```python
from build123d import *

# Parameters (mm, degrees)
BOSS_EXTRUDE1_DEPTH = 4.5
FILLET1_R           = 0.3
FILLET2_R           = 0.3
SHELL3_START        = 0.35
SHELL3_DEPTH        = 3.8
SKETCH3_W           = 12.9
SKETCH3_H           = 3.9
CUT_EXTRUDE1_DEPTH  = 21
CUT_EXTRUDE2_REACH  = 27.289
SKETCH4_W           = 3
SKETCH4_H           = 2.5


# Read off the part's stored shape, not the designer's step: Shell3
with BuildPart() as part:
    # Sketch1 → Boss-Extrude1 (new body)
    with BuildSketch(Plane(origin=(0, 0, 0), x_dir=(1, 0, 0), z_dir=(0, 1, 0))):
        Polygon((-6.75, -7.047619048), (6.75, -7.047619048), (6.75, 13.952380952), (6, 15.365710355), (6, 23.952380952), (-6, 23.952380952), (-6, 15.365710355), (-6.75, 13.952380952), align=None)
    extrude(amount=BOSS_EXTRUDE1_DEPTH)

    # Fillet1
    fillet1_edges = [part.edges().sort_by_distance(p)[0] for p in [
        (6, 4.5, -19.659045654),
        (6.375, 0, -14.659045654),
        (6.75, 0, -3.452380952),
        (0, 4.5, -23.952380952),
        (-6, 4.5, -19.659045654),
        (-6.375, 4.5, -14.659045654),
        (-6.75, 4.5, -3.452380952),
        (0, 4.5, 7.047619048),
        (6.75, 4.5, -3.452380952),
        (6.375, 4.5, -14.659045654),
        (0, 0, 7.047619048),
        (-6.75, 0, -3.452380952),
        (-6.375, 0, -14.659045654),
        (-6, 0, -19.659045654),
        (0, 0, -23.952380952),
        (6, 0, -19.659045654),
    ]]
    fillet(fillet1_edges, radius=FILLET1_R)

    # Fillet2
    # the kernel refuses this fillet: 0.3 mm, written as the material it takes off along each edge
    with BuildSketch(Plane(origin=(-6.45, 0.3, 6.747619048), x_dir=(-1, 0, 0), z_dir=(0, 0, 1))) as fillet2_piece_1_section:
        Polygon((0, 0), (FILLET2_R, 0), (FILLET2_R, FILLET2_R), (0, FILLET2_R), align=None)
    fillet2_piece_1 = extrude(amount=FILLET2_R, mode=Mode.PRIVATE)
    fillet2_piece_1 = fillet2_piece_1 - Plane(origin=(-6.45, 0.3, 6.747619048), x_dir=(0.7071067811865475, 0.7071067811865475, 0), z_dir=(0, 0, 1)) * Sphere(FILLET2_R, mode=Mode.PRIVATE)
    add(fillet2_piece_1, mode=Mode.SUBTRACT)
    with BuildSketch(Plane(origin=(-5.7, 0.3, -23.652380952), x_dir=(0, 0, -1), z_dir=(-1, 0, 0))) as fillet2_piece_2_section:
        Polygon((0, 0), (FILLET2_R, 0), (FILLET2_R, FILLET2_R), (0, FILLET2_R), align=None)
    fillet2_piece_2 = extrude(amount=FILLET2_R, mode=Mode.PRIVATE)
    fillet2_piece_2 = fillet2_piece_2 - Plane(origin=(-5.7, 0.3, -23.652380952), x_dir=(0, 0.7071067811865475, 0.7071067811865475), z_dir=(-1, 0, 0)) * Sphere(FILLET2_R, mode=Mode.PRIVATE)
    add(fillet2_piece_2, mode=Mode.SUBTRACT)
    with BuildSketch(Plane(origin=(6.45, 0.3, 6.747619048), x_dir=(1, 0, 0), z_dir=(0, 0, 1))) as fillet2_piece_3_section:
        Polygon((0, 0), (FILLET2_R, 0), (FILLET2_R, -FILLET2_R), (0, -FILLET2_R), align=None)
    fillet2_piece_3 = extrude(amount=FILLET2_R, mode=Mode.PRIVATE)
    fillet2_piece_3 = fillet2_piece_3 - Plane(origin=(6.45, 0.3, 6.747619048), x_dir=(-0.7071067811865475, 0.7071067811865475, 0), z_dir=(0, 0, 1)) * Sphere(FILLET2_R, mode=Mode.PRIVATE)
    add(fillet2_piece_3, mode=Mode.SUBTRACT)
    with BuildSketch(Plane(origin=(5.7, 0.3, -23.652380952), x_dir=(0, 0, -1), z_dir=(1, 0, 0))) as fillet2_piece_4_section:
        Polygon((0, 0), (FILLET2_R, 0), (FILLET2_R, -FILLET2_R), (0, -FILLET2_R), align=None)
    fillet2_piece_4 = extrude(amount=FILLET2_R, mode=Mode.PRIVATE)
    fillet2_piece_4 = fillet2_piece_4 - Plane(origin=(5.7, 0.3, -23.652380952), x_dir=(0, 0.7071067811865475, 0.7071067811865475), z_dir=(1, 0, 0)) * Sphere(FILLET2_R, mode=Mode.PRIVATE)
    add(fillet2_piece_4, mode=Mode.SUBTRACT)
    with BuildSketch(Plane(origin=(-5.7, 4.2, -23.652380952), x_dir=(0, 0, -1), z_dir=(-1, 0, 0))) as fillet2_piece_5_section:
        Polygon((0, 0), (FILLET2_R, 0), (FILLET2_R, -FILLET2_R), (0, -FILLET2_R), align=None)
    fillet2_piece_5 = extrude(amount=FILLET2_R, mode=Mode.PRIVATE)
    fillet2_piece_5 = fillet2_piece_5 - Plane(origin=(-5.7, 4.2, -23.652380952), x_dir=(0, -0.7071067811865475, 0.7071067811865475), z_dir=(-1, 0, 0)) * Sphere(FILLET2_R, mode=Mode.PRIVATE)
    add(fillet2_piece_5, mode=Mode.SUBTRACT)
    with BuildSketch(Plane(origin=(5.7, 4.2, -23.652380952), x_dir=(0, 0, -1), z_dir=(1, 0, 0))) as fillet2_piece_6_section:
        Polygon((0, 0), (FILLET2_R, 0), (FILLET2_R, FILLET2_R), (0, FILLET2_R), align=None)
    fillet2_piece_6 = extrude(amount=FILLET2_R, mode=Mode.PRIVATE)
    fillet2_piece_6 = fillet2_piece_6 - Plane(origin=(5.7, 4.2, -23.652380952), x_dir=(0, -0.7071067811865475, 0.7071067811865475), z_dir=(1, 0, 0)) * Sphere(FILLET2_R, mode=Mode.PRIVATE)
    add(fillet2_piece_6, mode=Mode.SUBTRACT)
    with BuildSketch(Plane(origin=(-6.45, 4.2, 6.747619048), x_dir=(-1, 0, 0), z_dir=(0, 0, 1))) as fillet2_piece_7_section:
        Polygon((0, 0), (FILLET2_R, 0), (FILLET2_R, -FILLET2_R), (0, -FILLET2_R), align=None)
    fillet2_piece_7 = extrude(amount=FILLET2_R, mode=Mode.PRIVATE)
    fillet2_piece_7 = fillet2_piece_7 - Plane(origin=(-6.45, 4.2, 6.747619048), x_dir=(0.7071067811865475, -0.7071067811865475, 0), z_dir=(0, 0, 1)) * Sphere(FILLET2_R, mode=Mode.PRIVATE)
    add(fillet2_piece_7, mode=Mode.SUBTRACT)
    with BuildSketch(Plane(origin=(6.45, 4.2, 6.747619048), x_dir=(1, 0, 0), z_dir=(0, 0, 1))) as fillet2_piece_8_section:
        Polygon((0, 0), (FILLET2_R, 0), (FILLET2_R, FILLET2_R), (0, FILLET2_R), align=None)
    fillet2_piece_8 = extrude(amount=FILLET2_R, mode=Mode.PRIVATE)
    fillet2_piece_8 = fillet2_piece_8 - Plane(origin=(6.45, 4.2, 6.747619048), x_dir=(-0.7071067811865475, -0.7071067811865475, 0), z_dir=(0, 0, 1)) * Sphere(FILLET2_R, mode=Mode.PRIVATE)
    add(fillet2_piece_8, mode=Mode.SUBTRACT)
    with BuildSketch(Plane(origin=(6, 0.3, -23.952380952), x_dir=(0, 0, 1), z_dir=(0, 1, 0)), Plane(origin=(6.75, 0.3, 7.047619048), x_dir=(-1, 0, 0), z_dir=(0, 1, 0))) as fillet2_piece_9:
        with BuildLine():
            CenterArc((FILLET2_R, -FILLET2_R), FILLET2_R, 90, 90)
            Line((0, -FILLET2_R), (0, 0))
            Line((0, 0), (FILLET2_R, 0))
        make_face()
    extrude(amount=3.9, mode=Mode.SUBTRACT)
    with BuildSketch(Plane(origin=(-6, 0.3, -23.952380952), x_dir=(0, 0, 1), z_dir=(0, 1, 0)), Plane(origin=(-6.75, 0.3, 7.047619048), x_dir=(1, 0, 0), z_dir=(0, 1, 0))) as fillet2_piece_10:
        with BuildLine():
            CenterArc((FILLET2_R, FILLET2_R), FILLET2_R, 180, 90)
            Line((0, FILLET2_R), (0, 0))
            Line((0, 0), (FILLET2_R, 0))
        make_face()
    extrude(amount=3.9, mode=Mode.SUBTRACT)

    # Shell3 outline → Shell3 (cut)
    with BuildSketch(Plane(origin=(0, 0, 0), x_dir=(1, 0, 0), z_dir=(0, 1, 0)).offset(SHELL3_START)):
        Polygon((6.4, -6.697619048), (6.4, 13.865268007), (5.65, 15.278597409), (5.65, 23.952380952), (-5.65, 23.952380952), (-5.65, 15.278597409), (-6.4, 13.865268007), (-6.4, -6.697619048), align=None)
    extrude(amount=SHELL3_DEPTH, mode=Mode.SUBTRACT)

    # Sketch3 → Cut-Extrude1 (cut)
    with BuildSketch(Plane.XY.offset(7.047619048)):
        with Locations((0, 2.25)):
            Rectangle(SKETCH3_W, SKETCH3_H)
    extrude(amount=-CUT_EXTRUDE1_DEPTH, mode=Mode.SUBTRACT)

    # Sketch4 → Cut-Extrude2 (cut, up to next)
    with BuildSketch(Plane(origin=(0, 4.5, 0), x_dir=(1, 0, 0), z_dir=(0, 1, 0)), mode=Mode.PRIVATE) as cut_extrude2_sk1:
        with Locations((3, 18.402380952)):
            Rectangle(SKETCH4_W, SKETCH4_H)
    cut_extrude2_tool1 = extrude(cut_extrude2_sk1.sketch, amount=-CUT_EXTRUDE2_REACH, mode=Mode.PRIVATE) & part.part
    # Sketch4 → Cut-Extrude2 (cut, up to next)
    with BuildSketch(Plane(origin=(0, 4.5, 0), x_dir=(1, 0, 0), z_dir=(0, 1, 0)), mode=Mode.PRIVATE) as cut_extrude2_sk2:
        with Locations((-3, 18.402380952)):
            Rectangle(SKETCH4_W, SKETCH4_H)
    cut_extrude2_tool2 = extrude(cut_extrude2_sk2.sketch, amount=-CUT_EXTRUDE2_REACH, mode=Mode.PRIVATE) & part.part
    add(cut_extrude2_tool1.solids().sort_by_distance((3, 4.5, -18.402381))[0], mode=Mode.SUBTRACT)
    add(cut_extrude2_tool2.solids().sort_by_distance((-3, 4.5, -18.402381))[0], mode=Mode.SUBTRACT)


solid = part.part
```
Source: CAD feature listing. Evaluate the final solid. Frame: model axes, mm. A direction names the side the tool comes from. Coordinates: 2 decimals unless noted, no trailing zeros. Write each loop counter-clockwise with the first axis right and the second up, starting at its lowest first coordinate (ties: lowest second). Pieces come first, ordered by that corner, then holes. Notation, with made-up numbers: (-19.75, -24) -> (36.25, -24) arc R11 ccw to (36.25, -19) -> close; hole circle Ø3 at (49.5, 54.5). An arc over 180 degrees is marked (long way). Return JSON: item names as keys, results as strings. Group by question number.
1) Ray query, line 1 along X through (y, z) = (2.8, -7); line 2 along Y through (x, z) = (-4.25, -5.5); line 3 along X through (y, z) = (1.25, -16). Return the intervals inside material, ascending.
2) Section query A-A, the plane y = 3.25. Return loops of the section in (x, z).
3) Mould query, pull axis Y, two halves, no side actions, for faces 6 (the face through (6.28, 4.41, -14.66)), 7 (the face through (-6, 2.22, -14.62)), 8 (the face through (0, 0, -9)). Classes: +Y half, -Y half, draft (parallel to the pull), parting line (faces both ways), or undercut.
4) Set-up query: faces 1 (the face through (-5.65, 2, -20)), 2 (the face through (-6.29, 4.41, -14.64)), 3 (the face through (6, 2, -19)), 4 (the face through (6.45, 2, -3)), 5 (the face through (-6.37, 2.22, -14.67)). Return all of +Z, -Z, +X, -X, +Y, -Y with unobstructed straight access to the full face (end or side cutting, diameter ignored); none if empty.
5) Section query B-B, the plane x = 2. Return loops of the section in (y, z), plus the area to 3 significant figures.
6) Contact query for flat-ended pins moving along their axis: P1, Ø1.9, axis at y = 2, z = -19, coming from the +X side; P2, Ø2, axis at y = 1.5, z = -18, coming from the -X side; P3, Ø2, axis at x = 1, y = 2, coming from the -Z side. Output: stop coordinate, or through.
7) Section query C-C, the plane z = -3.5. Return loops of the section in (x, y).
8) Section query D-D, the plane z = -21.5. Return loops of the section in (x, y), plus the area to 3 significant figures.
From the geometry:
{
 "1": {"line 1": "-6.75 to -6.45, 6.45 to 6.75", "line 2": "0 to 0.3, 4.2 to 4.5", "line 3": "-6 to -5.65, 5.65 to 6"},
 "2": {"outline": "(-6.75, -13.95) -> (-6, -15.37) -> (-6, -23.65) arc R0.3 ccw to (-5.7, -23.95) -> (-5.65, -23.95) -> (-5.65, -15.28) -> (-6.35, -13.95) -> (-6.45, -13.95) -> (-6.45, 7.05) arc R0.3 ccw to (-6.75, 6.75) -> close; (5.65, -23.95) -> (5.7, -23.95) arc R0.3 ccw to (6, -23.65) -> (6, -15.37) -> (6.75, -13.95) -> (6.75, 6.75) arc R0.3 ccw to (6.45, 7.05) -> (6.45, -13.95) -> (6.35, -13.95) -> (5.65, -15.28) -> close"},
 "3": {"face 6": "+Y half", "face 7": "undercut", "face 8": "-Y half"},
 "4": {"face 1": "+Z, -Z", "face 2": "-Z, -X, +Y", "face 3": "-Z, +X, +Y, -Y", "face 4": "+Z", "face 5": "-Z, -X, +Y, -Y"},
 "5": {"outline": "(0, -23.65) arc R0.3 ccw to (0.3, -23.95) -> (0.35, -23.95) -> (0.35, -13.95) -> (0.3, -13.95) -> (0.3, 7.05) arc R0.3 ccw to (0, 6.75) -> close; (4.15, -23.95) -> (4.2, -23.95) arc R0.3 ccw to (4.5, -23.65) -> (4.5, -19.65) -> (4.15, -19.65) -> close; (4.15, -17.15) -> (4.5, -17.15) -> (4.5, 6.75) arc R0.3 ccw to (4.2, 7.05) -> (4.2, -13.95) -> (4.15, -13.95) -> close", "area": "18.6 mm²"},
 "6": {"P1": "x = 6", "P2": "x = -6", "P3": "through"},
 "7": {"outline": "(-6.75, 0.3) arc R0.3 ccw to (-6.45, 0) -> (6.45, 0) arc R0.3 ccw to (6.75, 0.3) -> (6.75, 4.2) arc R0.3 ccw to (6.45, 4.5) -> (-6.45, 4.5) arc R0.3 ccw to (-6.75, 4.2) -> close; hole (-6.45, 0.3) -> (6.45, 0.3) -> (6.45, 4.2) -> (-6.45, 4.2) -> close"},
 "8": {"outline": "(-6, 0.3) arc R0.3 ccw to (-5.7, 0) -> (5.7, 0) arc R0.3 ccw to (6, 0.3) -> (6, 4.2) arc R0.3 ccw to (5.7, 4.5) -> (-5.7, 4.5) arc R0.3 ccw to (-6, 4.2) -> close; hole (-5.65, 0.35) -> (5.65, 0.35) -> (5.65, 4.15) -> (-5.65, 4.15) -> close", "area": "11.0 mm²"}
}
